Study the drawing (mm; zero at the part's minimum x, y, z) and answer. Coordinates: 2 decimals unless noted, no trailing zeros. Loops run counter-clockwise (first coordinate to the right, second up) from the corner with the lowest first, then second, coordinate; pieces in that order, holes last. Notation, with made-up numbers: (37.25, -16) - (45.25, -16) arc R38 cw to (45.25, 23) - close; hole circle Ø6 at (-16.5, 14.25). An arc over 180 degrees is marked (long way). Write each question's results on one line, items separated by ' | '. Start each with the question number.
(1) Find section A-A on z = 9.75. Determine the outline of the cut face in (x, y), then the cut area to 3 significant figures.
(2) Find section B-B on x = 6.5. State how many separate pieces and enclosed holes the cut face has, then the cut area to 4 significant figures.
(3) Given pin 1 Ø2 at (x, z) = (6.5, 8) entering from +Y, flat-ended and moving along its own axis, determine where the tip first touches the part or whether it passes through.
(4) Determine the mould class of the marked faces 1, 2 and 3 for opening direction Y: released by +Y, released by -Y, zero draft, split by the parting line, or undercut.
(5) Find section C-C on z = 12.5. Determine the outline of the cut face in (x, y).
(6) Find section D-D on y = 16. Determine the outline of the cut face in (x, z).
(7) Consider line 1 (X direction, y = 8.5, z = 3); line 2 (Y direction, x = 4, z = 13.25); line 3 (Y direction, x = 3, z = 15). Determine where each line is inside the solid, lowest interval first. Write a range as from..to.
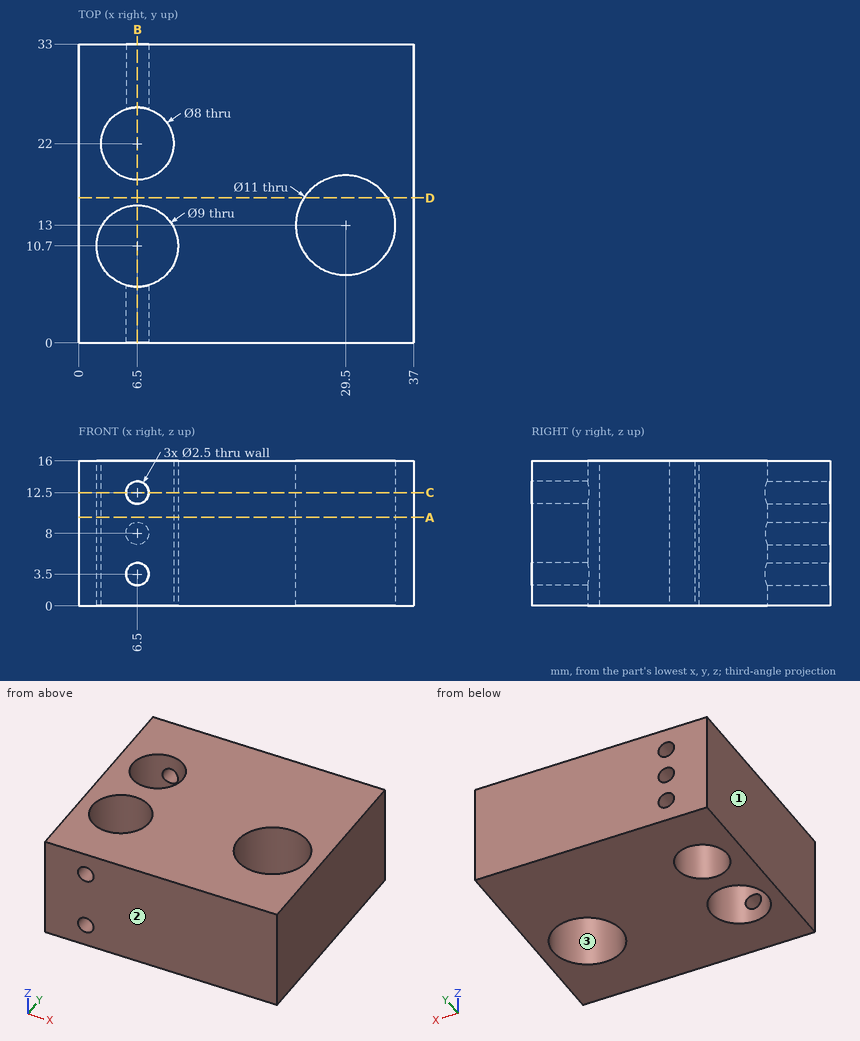
Values:
1) outline: (0, 0) - (37, 0) - (37, 33) - (0, 33) - close; hole circle Ø9 at (6.5, 10.7); hole circle Ø8 at (6.5, 22); hole circle Ø11 at (29.5, 13) | area: 1,010 mm²
2) separate pieces: 8 | enclosed holes: 0 | area: 172.5 mm²
3) pin 1: stops at y = 18.13
4) face 1: zero draft | face 2: released by -Y | face 3: undercut
5) outline: (0, 0) - (5.25, 0) - (5.25, 6.38) arc R4.5 cw (long way) to (7.75, 6.38) - (7.75, 0) - (37, 0) - (37, 33) - (7.75, 33) - (7.75, 25.8) arc R4 cw (long way) to (5.25, 25.8) - (5.25, 33) - (0, 33) - close; hole circle Ø11 at (29.5, 13)
6) outline: (0, 0) - (24.89, 0) - (24.89, 16) - (0, 16) - close; (34.11, 0) - (37, 0) - (37, 16) - (34.11, 16) - close
7) line 1: x = 0..2.57, 10.43..26.34, 32.66..37 | line 2: y = 0..6.96, 14.44..18.88, 25.12..33 | line 3: y = 0..7.87, 13.53..20.06, 23.94..33
